from build123d import *

# Parameters (mm, degrees)
EXTRUDE_1_DEPTH       = 2
HOLE_WIZARD_M81_D     = 8.4
HOLE_WIZARD_M81_DEPTH = 2
CHAMFER_1_SIZE        = 2


with BuildPart() as part:
    # Эскиз1 → Бобышка-Вытянуть1 (new body)
    with BuildSketch(Plane(origin=(0, 0, 0), x_dir=(1, 0, 0), z_dir=(0, 0, -1))):
        Polygon((0, 0), (0, 180), (90, 180), (90, 90), (45, 0), align=None)
    extrude(amount=EXTRUDE_1_DEPTH)

    # Отверстие с зазором M81
    with Locations(Plane(origin=(0, 0, -2), x_dir=(1, 0, 0), z_dir=(0, 0, -1))):
        with Locations((22.5, 157.5), (22.5, 112.5), (22.5, 67.5), (22.5, 22.5), (67.5, 157.5), (67.5, 112.5)):
            Hole(HOLE_WIZARD_M81_D / 2, depth=HOLE_WIZARD_M81_DEPTH)

    # Фаска1
    chamfer_1_edges = [part.edges().sort_by_distance(p)[0] for p in [
        (0, 0, -1),
        (0, -180, -1),
        (90, -180, -1),
    ]]
    chamfer(chamfer_1_edges, length=CHAMFER_1_SIZE)


solid = part.part
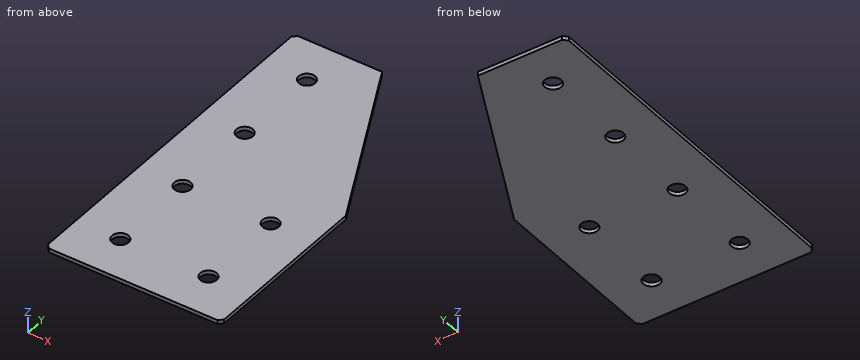
CAD build for the part. Positions are in the model's coordinates, mm. Round coordinates to 2 decimals unless told otherwise and drop trailing zeros. Order: outer loops, then holes, each group sorted by start corner. A loop starts at its lowest first (then second) coordinate and runs counter-clockwise, first axis right, second up. Notation, with made-up numbers: (-9, -33.75) -> (9, -33.75) arc R17 ccw to (9, -9.75) -> close; hole circle Ø11 at (79, 61.25). An arc over 180 degrees is marked (long way). Write each question's results on one line, items separated by ' | '.
1. Wall check: line 1 along Y through (x, z) = (22.5, -1); line 2 along X through (y, z) = (-157.5, -1); line 3 along X through (y, z) = (-22.5, -0.55). Give the ranges that are in metal, low to high. Write a range as [from, to].
Findings below:
line 1: y = [-180, -161.7], [-153.3, -116.7], [-108.3, -71.7], [-63.3, -26.7], [-18.3, 0] | line 2: x = [0, 18.3], [26.7, 63.3], [71.7, 90] | line 3: x = [0, 18.3], [26.7, 56.25]
2. Cut at B-B (y = -67.5). Give the cut face in (x, z), plus the area to 3 significant figures.
Findings below:
outline: (0, -2) -> (18.3, -2) -> (18.3, 0) -> (0, 0) -> close; (26.7, -2) -> (78.75, -2) -> (78.75, 0) -> (26.7, 0) -> close | area: 141 mm²
3. Cut at D-D (x = 22.5). Give the cut face in (y, z), plus the area to 3 significant figures.
Findings below:
outline: (-180, -2) -> (-161.7, -2) -> (-161.7, 0) -> (-180, 0) -> close; (-153.3, -2) -> (-116.7, -2) -> (-116.7, 0) -> (-153.3, 0) -> close; (-108.3, -2) -> (-71.7, -2) -> (-71.7, 0) -> (-108.3, 0) -> close; (-63.3, -2) -> (-26.7, -2) -> (-26.7, 0) -> (-63.3, 0) -> close; (-18.3, -2) -> (0, -2) -> (0, 0) -> (-18.3, 0) -> close | area: 293 mm²
4. Cut at C-C (z = -1.6). Give the cut face in (x, y).
Findings below:
outline: (0, -178) -> (2, -180) -> (88, -180) -> (90, -178) -> (90, -90) -> (45, 0) -> (2, 0) -> (0, -2) -> close; hole circle Ø8.4 at (22.5, -157.5); hole circle Ø8.4 at (22.5, -112.5); hole circle Ø8.4 at (22.5, -67.5); hole circle Ø8.4 at (22.5, -22.5); hole circle Ø8.4 at (67.5, -157.5); hole circle Ø8.4 at (67.5, -112.5)
5. Cut at A-A (x = 67.5). Give the cut face in (y, z).
Findings below:
outline: (-180, -2) -> (-161.7, -2) -> (-161.7, 0) -> (-180, 0) -> close; (-153.3, -2) -> (-116.7, -2) -> (-116.7, 0) -> (-153.3, 0) -> close; (-108.3, -2) -> (-45, -2) -> (-45, 0) -> (-108.3, 0) -> close
